Geometry: final body of the model. Coordinates: model frame, mm. Round coordinates to 2 decimals unless told otherwise and drop trailing zeros. Order: outer loops, then holes, each group sorted by start corner. A loop starts at its lowest first (then second) coordinate and runs counter-clockwise, first axis right, second up. Notation, with made-up numbers: M -9,-15 L 7,-15 A22 ccw 7,-1 Z; hole C 13,-37 d9. An arc over 180 degrees is marked long. Put each result on its own line as item: value. Start each with the question number.
1) First-contact query: P1, Ø5, axis at y = 713, z = 41.5, coming from the +X side; P2, Ø4, axis at y = 828, z = 15.5, coming from the +X side. Flat tips, straight axial feed; report the tip coordinate or a pass-through.
2) Material intervals for probe 1 along Z at (x, y) = (53, 485.5); probe 2 along X at (y, z) = (412.5, 83); probe 3 along Z at (x, y) = (26.5, 1011), sorted ascending. Write a range as [from, to].
3) Section A-A, the plane y = 810. Return loops of the section in (x, z).
4) Section B-B, the plane z = 63.5. Return loops of the section in (x, y), then the cut area to 3 significant figures.
5) Section C-C, the plane x = 96. Return loops of the section in (y, z).
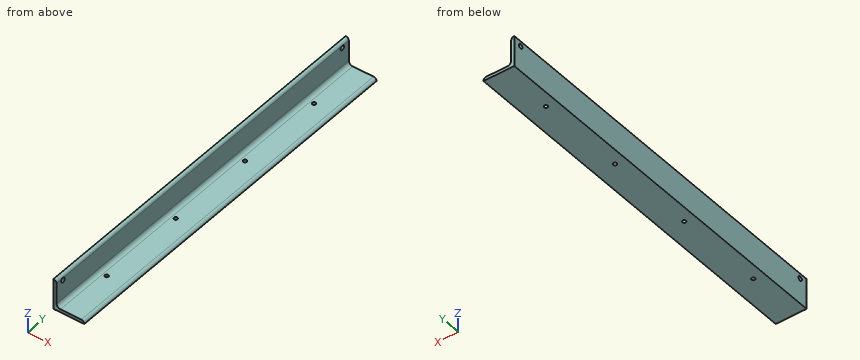
from build123d import *

# Parameters (mm, degrees)
F2_DEPTH = 1480
F4_D     = 17.5
F6_D     = 13.5


with BuildPart() as f2:
    # F1 (on Front) → F2 (new body)
    with BuildSketch(Plane.XZ):
        with BuildLine():
            Line((0, 120), (0, 0))
            Line((0, 0), (120, 0))
            ThreePointArc((120, 0), (116.6491099907, 8.3182267562), (108.4678506053, 11.9908763571))
            Line((108.4678506053, 11.9908763571), (27.0373860807, 12.047892481))
            ThreePointArc((27.0373860807, 12.047892481), (16.4412870863, 16.4412870863), (12.047892481, 27.0373860807))
            Line((12.047892481, 27.0373860807), (11.9908763571, 108.4678506053))
            ThreePointArc((11.9908763571, 108.4678506053), (8.3182267562, 116.6491099907), (0, 120))
        make_face()
    extrude(amount=-F2_DEPTH)

    # F4 (through all)
    with Locations(Plane(origin=(12.0668176491, 0, 0.0084489653), x_dir=(0, 1, 0), z_dir=(0.9999997549, 0, 0.0007001816))):
        with Locations((32.5, 100), (1447.5, 100)):
            Hole(F4_D / 2)

    # F6 (through all)
    with Locations(Plane(origin=(0.0084489653, 0, 12.0668176491), x_dir=(0.9999997549, 0, -0.0007001816), z_dir=(0.0007001816, 0, 0.9999997549))):
        with Locations((42.0289584485, 215), (42.0289584485, 565), (42.0289584485, 915), (42.0289584485, 1265)):
            Hole(F6_D / 2)


solid = f2.part
Result sheet:
1. P1: stops at x = 12.04
1. P2: stops at x = 20.61
2. probe 1: z = [0, 12.03]
2. probe 2: x = [0, 12.01]
2. probe 3: z = [0, 12.06]
3. outline: M 0,0 L 120,0 A12 ccw 108.47,11.99 L 27.04,12.05 A15 cw 12.05,27.04 L 11.99,108.47 A12 ccw 0,120 Z
4. outline: M 0,0 L 12.02,0 L 12.02,1480 L 0,1480 Z
4. area: 17,800 mm2
5. outline: M 0,0 L 1480,0 L 1480,12 L 0,12 Z
